Input: part model. Units: mm. Frame: model coordinates. A direction names the side the tool comes from. Give positions to 0.01 mm unless a question says otherwise; leave off trailing zeros. Loops run counter-clockwise (first coordinate to the right, second up) from the corner with the lowest first, then second, coordinate; pieces in that order, holes last. Notation, with made-up numbers: (87, -13.75) -> (107, -13.75) arc R24 cw to (107, 16.25) -> close; hole circle Ø11 at (68.25, -35.5). An arc over 180 degrees is marked (long way). Use CSV: the item, a comma, the result in double quotes.
```python
from build123d import *

# Parameters (mm, degrees)
BOX743_W                     = 30.2
BOX743_H                     = 30.2
BOX743_DEPTH                 = 25
CYLINDER1930_R               = 1.5
CYLINDER1930_DEPTH           = 20
CYLINDER1930_PLACEMENT_ANGLE = 45
CYLINDER1927_R               = 1.5
CYLINDER1927_DEPTH           = 20
CYLINDER1933_R               = 1.5
CYLINDER1933_DEPTH           = 20
CYLINDER1933_PLACEMENT_ANGLE = 135
CYLINDER1929_R               = 1.5
CYLINDER1929_DEPTH           = 20
CYLINDER1935_R               = 1.5
CYLINDER1935_DEPTH           = 20
CYLINDER1935_PLACEMENT_ANGLE = 225
CYLINDER1928_R               = 1.5
CYLINDER1928_DEPTH           = 20
CYLINDER1943_R               = 1.5
CYLINDER1943_DEPTH           = 20
CYLINDER1943_PLACEMENT_ANGLE = 45
CYLINDER1937_R               = 1.5
CYLINDER1937_DEPTH           = 20
CYLINDER1940_R               = 3
CYLINDER1940_DEPTH           = 3
CYLINDER1940_PLACEMENT_ANGLE = 45
CYLINDER1942_R               = 3
CYLINDER1942_DEPTH           = 3
CYLINDER1941_R               = 3
CYLINDER1941_DEPTH           = 3
CYLINDER1941_PLACEMENT_ANGLE = 135
CYLINDER1939_R               = 3
CYLINDER1939_DEPTH           = 3
CYLINDER1932_R               = 3
CYLINDER1932_DEPTH           = 3
CYLINDER1932_PLACEMENT_ANGLE = 225
CYLINDER1938_R               = 3
CYLINDER1938_DEPTH           = 3
CYLINDER1931_R               = 3
CYLINDER1931_DEPTH           = 3
CYLINDER1931_PLACEMENT_ANGLE = 45
CYLINDER1934_R               = 3
CYLINDER1934_DEPTH           = 3
CYLINDER1936_R               = 34
CYLINDER1936_DEPTH           = 6
CHAMFER078_SIZE              = 0.5


with BuildPart() as krychle743:
    # Box743 → Box743 (new body)
    with BuildSketch(Plane(origin=(-15.1, -15.1, 0), x_dir=(1, 0, 0), z_dir=(0, 0, 1))):
        with Locations((15.1, 15.1)):
            Rectangle(BOX743_W, BOX743_H)
    extrude(amount=BOX743_DEPTH)


with BuildPart() as obj1:
    # Cylinder1930 → Cylinder1930 (new body)
    with BuildSketch(Plane.XY):
        Circle(CYLINDER1930_R)
    extrude(amount=CYLINDER1930_DEPTH)


with BuildPart() as obj1_1:
    # Cylinder1930 placement: moved
    add(obj1.part.moved(Location((-18.031223, 18.031223, -4))).rotate(Axis((-18.031223, 18.031223, -4), (0, 0, 1)), CYLINDER1930_PLACEMENT_ANGLE))


with BuildPart() as obj2:
    # Cylinder1927 → Cylinder1927 (new body)
    with BuildSketch(Plane(origin=(-25.5, 0, -4), x_dir=(0, 1, 0), z_dir=(0, 0, 1))):
        Circle(CYLINDER1927_R)
    extrude(amount=CYLINDER1927_DEPTH)


with BuildPart() as obj3:
    # Cylinder1933 → Cylinder1933 (new body)
    with BuildSketch(Plane.XY):
        Circle(CYLINDER1933_R)
    extrude(amount=CYLINDER1933_DEPTH)


with BuildPart() as obj3_1:
    # Cylinder1933 placement: moved
    add(obj3.part.moved(Location((-18.031223, -18.031223, -4))).rotate(Axis((-18.031223, -18.031223, -4), (0, 0, 1)), CYLINDER1933_PLACEMENT_ANGLE))


with BuildPart() as obj4:
    # Cylinder1929 → Cylinder1929 (new body)
    with BuildSketch(Plane(origin=(0, -25.5, -4), x_dir=(-1, 0, 0), z_dir=(0, 0, 1))):
        Circle(CYLINDER1929_R)
    extrude(amount=CYLINDER1929_DEPTH)


with BuildPart() as obj5:
    # Cylinder1935 → Cylinder1935 (new body)
    with BuildSketch(Plane.XY):
        Circle(CYLINDER1935_R)
    extrude(amount=CYLINDER1935_DEPTH)


with BuildPart() as obj5_1:
    # Cylinder1935 placement: moved
    add(obj5.part.moved(Location((18.031223, -18.031223, -4))).rotate(Axis((18.031223, -18.031223, -4), (0, 0, 1)), CYLINDER1935_PLACEMENT_ANGLE))


with BuildPart() as obj6:
    # Cylinder1928 → Cylinder1928 (new body)
    with BuildSketch(Plane(origin=(25.5, 0, -4), x_dir=(0, -1, 0), z_dir=(0, 0, 1))):
        Circle(CYLINDER1928_R)
    extrude(amount=CYLINDER1928_DEPTH)


with BuildPart() as obj7:
    # Cylinder1943 → Cylinder1943 (new body)
    with BuildSketch(Plane.XY):
        Circle(CYLINDER1943_R)
    extrude(amount=CYLINDER1943_DEPTH)


with BuildPart() as obj7_1:
    # Cylinder1943 placement: moved
    add(obj7.part.moved(Location((18.031223, 18.031223, -4))).rotate(Axis((18.031223, 18.031223, -4), (0, 0, -1)), CYLINDER1943_PLACEMENT_ANGLE))


with BuildPart() as compound919:
    # Cylinder1937 → Cylinder1937 (new body)
    with BuildSketch(Plane(origin=(0, 25.5, -4), x_dir=(1, 0, 0), z_dir=(0, 0, 1))):
        Circle(CYLINDER1937_R)
    extrude(amount=CYLINDER1937_DEPTH)

    # Compound919: union obj1, obj2, obj3, obj4, obj5, obj6, obj7
    add(obj1_1.part)
    add(obj2.part)
    add(obj3_1.part)
    add(obj4.part)
    add(obj5_1.part)
    add(obj6.part)
    add(obj7_1.part)


with BuildPart() as obj8:
    # Cylinder1940 → Cylinder1940 (new body)
    with BuildSketch(Plane.XY):
        Circle(CYLINDER1940_R)
    extrude(amount=CYLINDER1940_DEPTH)


with BuildPart() as obj8_1:
    # Cylinder1940 placement: moved
    add(obj8.part.moved(Location((-18.031223, 18.031223, 3))).rotate(Axis((-18.031223, 18.031223, 3), (0, 0, 1)), CYLINDER1940_PLACEMENT_ANGLE))


with BuildPart() as obj9:
    # Cylinder1942 → Cylinder1942 (new body)
    with BuildSketch(Plane(origin=(-25.5, 0, 3), x_dir=(0, 1, 0), z_dir=(0, 0, 1))):
        Circle(CYLINDER1942_R)
    extrude(amount=CYLINDER1942_DEPTH)


with BuildPart() as obj10:
    # Cylinder1941 → Cylinder1941 (new body)
    with BuildSketch(Plane.XY):
        Circle(CYLINDER1941_R)
    extrude(amount=CYLINDER1941_DEPTH)


with BuildPart() as obj10_1:
    # Cylinder1941 placement: moved
    add(obj10.part.moved(Location((-18.031223, -18.031223, 3))).rotate(Axis((-18.031223, -18.031223, 3), (0, 0, 1)), CYLINDER1941_PLACEMENT_ANGLE))


with BuildPart() as obj11:
    # Cylinder1939 → Cylinder1939 (new body)
    with BuildSketch(Plane(origin=(0, -25.5, 3), x_dir=(-1, 0, 0), z_dir=(0, 0, 1))):
        Circle(CYLINDER1939_R)
    extrude(amount=CYLINDER1939_DEPTH)


with BuildPart() as obj12:
    # Cylinder1932 → Cylinder1932 (new body)
    with BuildSketch(Plane.XY):
        Circle(CYLINDER1932_R)
    extrude(amount=CYLINDER1932_DEPTH)


with BuildPart() as obj12_1:
    # Cylinder1932 placement: moved
    add(obj12.part.moved(Location((18.031223, -18.031223, 3))).rotate(Axis((18.031223, -18.031223, 3), (0, 0, 1)), CYLINDER1932_PLACEMENT_ANGLE))


with BuildPart() as obj13:
    # Cylinder1938 → Cylinder1938 (new body)
    with BuildSketch(Plane(origin=(25.5, 0, 3), x_dir=(0, -1, 0), z_dir=(0, 0, 1))):
        Circle(CYLINDER1938_R)
    extrude(amount=CYLINDER1938_DEPTH)


with BuildPart() as obj14:
    # Cylinder1931 → Cylinder1931 (new body)
    with BuildSketch(Plane.XY):
        Circle(CYLINDER1931_R)
    extrude(amount=CYLINDER1931_DEPTH)


with BuildPart() as obj14_1:
    # Cylinder1931 placement: moved
    add(obj14.part.moved(Location((18.031223, 18.031223, 3))).rotate(Axis((18.031223, 18.031223, 3), (0, 0, -1)), CYLINDER1931_PLACEMENT_ANGLE))


with BuildPart() as compound918:
    # Cylinder1934 → Cylinder1934 (new body)
    with BuildSketch(Plane(origin=(0, 25.5, 3), x_dir=(1, 0, 0), z_dir=(0, 0, 1))):
        Circle(CYLINDER1934_R)
    extrude(amount=CYLINDER1934_DEPTH)

    # Compound918: union obj8, obj9, obj10, obj11, obj12, obj13, obj14
    add(obj8_1.part)
    add(obj9.part)
    add(obj10_1.part)
    add(obj11.part)
    add(obj12_1.part)
    add(obj13.part)
    add(obj14_1.part)


with BuildPart() as chamfer078:
    # Cylinder1936 → Cylinder1936 (new body)
    with BuildSketch(Plane.XY):
        Circle(CYLINDER1936_R)
    extrude(amount=CYLINDER1936_DEPTH)

    # Cut565: cut Compound918
    add(compound918.part, mode=Mode.SUBTRACT)

    # Cut566: cut Compound919
    add(compound919.part, mode=Mode.SUBTRACT)

    # Cut568: cut Krychle743
    add(krychle743.part, mode=Mode.SUBTRACT)

    # Chamfer078
    chamfer078_edges = [chamfer078.edges().sort_by_distance(p)[0] for p in [
        (-15.1, 0, 0),
        (0, -15.1, 0),
        (15.1, 0, 0),
        (0, 15.1, 0),
    ]]
    chamfer(chamfer078_edges, length=CHAMFER078_SIZE)


solid = chamfer078.part
```
1) Ray query, line 1 (Y direction, x = 19.5, z = 3.5); line 2 (Y direction, x = 12, z = 2.5); line 3 (Y direction, x = -25.5, z = 4). Return the intervals inside material, ascending.
From the geometry:
line 1,"y = -27.85 to -20.65, -15.42 to 15.42, 20.65 to 27.85"
line 2,"y = -31.81 to -15.1, 15.1 to 31.81"
line 3,"y = -22.49 to -3, 3 to 22.49"
2) Contact query for flat-ended pins moving along their axis: pin 1 (5 mm diameter, centred on x = -18.03, y = -18.03, fed in from +Z); pin 2 (1.5 mm diameter, centred on x = 21, z = 5, fed in from -Y); pin 3 (3 mm diameter, centred on y = 3, z = 2, fed in from +X). Output: stop coordinate, or through.
From the geometry:
pin 1,"stops at z = 3"
pin 2,"stops at y = -27.31"
pin 3,"stops at x = 33.97"
3) Section query B-B (y = -12). Return loops of the section in (x, z).
From the geometry:
outline,"(-31.81, 0) -> (-15.6, 0) -> (-15.1, 0.5) -> (-15.1, 6) -> (-31.81, 6) -> close; (15.1, 0.5) -> (15.6, 0) -> (31.81, 0) -> (31.81, 6) -> (15.1, 6) -> close"
4) Section query D-D (z = 4.5). Give the number of separate pieces and of enclosed holes in the cut face, then the cut area to 3 significant figures.
From the geometry:
separate pieces,"1"
enclosed holes,"9"
area,"2,490 mm^2"
5) Reachability of faces 1 (the cylindrical face through (19.86, 20.41, 4.48)), 2 (the flat face through (0, 15.1, 3)) from +Z, -Z, +X, -X, +Y, -Y: full face, straight path, thin tool, end or side. Return the list, or none.
From the geometry:
face 1,"+Z"
face 2,"+Z, -Z"
6) Section query C-C (x = 25.5). Return loops of the section in (y, z), then the cut area to 3 significant figures.
From the geometry:
outline,"(-22.49, 0) -> (-1.5, 0) -> (-1.5, 3) -> (-3, 3) -> (-3, 6) -> (-22.49, 6) -> close; (1.5, 0) -> (22.49, 0) -> (22.49, 6) -> (3, 6) -> (3, 3) -> (1.5, 3) -> close"
area,"243 mm^2"
7) Section query A-A (x = 0). Return loops of the section in (y, z), then the cut area to 3 significant figures.
From the geometry:
outline,"(-34, 0) -> (-27, 0) -> (-27, 3) -> (-28.5, 3) -> (-28.5, 6) -> (-34, 6) -> close; (-24, 0) -> (-15.6, 0) -> (-15.1, 0.5) -> (-15.1, 6) -> (-22.5, 6) -> (-22.5, 3) -> (-24, 3) -> close; (15.1, 0.5) -> (15.6, 0) -> (24, 0) -> (24, 3) -> (22.5, 3) -> (22.5, 6) -> (15.1, 6) -> close; (27, 0) -> (34, 0) -> (34, 6) -> (28.5, 6) -> (28.5, 3) -> (27, 3) -> close"
area,"173 mm^2"
